from build123d import *

# Parameters (mm, degrees)
BOSS_EXTRUDE1_DEPTH = 7
CUT_EXTRUDE1_DEPTH  = 8
CUT_EXTRUDE2_DEPTH  = 7
SKETCH5_R           = 1.25
CUT_EXTRUDE3_DEPTH  = 8
CUT_EXTRUDE4_DEPTH  = 8


with BuildPart() as part:
    # Sketch1 → Boss-Extrude1 (new body)
    with BuildSketch(Plane.XY):
        Polygon((0, 0), (10, 0), (10, 5), (40, 5), (47.5, -5), (55, -5), (62.5, 5), (55, 12.11693675), (47.5, 12.11693675), (32.5, 12.11693675), (0, 8.5), (0, 5), align=None)
    extrude(amount=BOSS_EXTRUDE1_DEPTH)

    # Sketch3 → Cut-Extrude1 (cut, through all)
    with BuildSketch(Plane.XY.offset(7)):
        Polygon((10, 5), (9.3, 0), (10, 0), align=None)
    extrude(amount=-CUT_EXTRUDE1_DEPTH, mode=Mode.SUBTRACT)

    # Sketch4 → Cut-Extrude2 (cut)
    with BuildSketch(Plane.XY.offset(7)):
        with BuildLine():
            ThreePointArc((51.468681491, 2.792101448), (46.488736675, 7.253317775), (40, 8.865334476))
            ThreePointArc((40, 8.865334476), (39, 7.865334476), (40, 6.865334476))
            ThreePointArc((40, 6.865334476), (45.552771274, 5.485842523), (49.814385807, 1.668132681))
            ThreePointArc((49.814385807, 1.668132681), (51.203518033, 1.402969222), (51.468681491, 2.792101448))
        make_face()
    extrude(amount=-CUT_EXTRUDE2_DEPTH, mode=Mode.SUBTRACT)

    # Sketch5 → Cut-Extrude3 (cut, through all)
    with BuildSketch(Plane.XY.offset(7)):
        with Locations((51.25, -2.5)):
            Circle(SKETCH5_R)
    extrude(amount=-CUT_EXTRUDE3_DEPTH, mode=Mode.SUBTRACT)

    # Sketch6 → Cut-Extrude4 (cut, through all)
    with BuildSketch(Plane.XY.offset(7)):
        Polygon((0, 0), (0.8, 0), (0, 5), align=None)
    extrude(amount=-CUT_EXTRUDE4_DEPTH, mode=Mode.SUBTRACT)


solid = part.part
For this review, take the finished solid that the model builds, in its own axes (mm). A direction names the side the tool comes from. Round coordinates to 2 decimals unless told otherwise and drop trailing zeros. Loops run counter-clockwise (first coordinate to the right, second up) from the corner with the lowest first, then second, coordinate; pieces in that order, holes last. Notation, with made-up numbers: (28.5, 76.25) - (39.5, 76.25) arc R20 ccw to (39.5, 85.25) - close; hole circle Ø7 at (17, 13). An arc over 180 degrees is marked (long way). Answer as CSV lines item,"result".
(1) Consider section B-B on z = 5. Give the boundary of the cut face in (x, y), then the cut area to 3 significant figures.
Checked values:
outline,"(0, 5) - (0.8, 0) - (9.3, 0) - (10, 5) - (40, 5) - (47.5, -5) - (55, -5) - (62.5, 5) - (55, 12.12) - (32.5, 12.12) - (0, 8.5) - close; hole (40, 6.87) arc R11.87 cw to (49.81, 1.67) arc R1 ccw to (51.47, 2.79) arc R13.87 ccw to (40, 8.87) arc R1 ccw to start; hole circle Ø2.5 at (51.25, -2.5)"
area,"522 mm2"
(2) Wall thickness on line 1 (Y direction, x = 51.25, z = 4.75); line 2 (Y direction, x = 38, z = 2.5); line 3 (Y direction, x = 43.5, z = 4.5): over which ranges is each line inside the solid? List them lowest first.
Checked values:
line 1,"y = -5 to -3.75, -1.25 to 1.44, 3.1 to 12.12"
line 2,"y = 5 to 12.12"
line 3,"y = 0.33 to 6.34, 8.42 to 12.12"
(3) Consider section D-D on y = 10.75. Give the boundary of the cut face in (x, z).
Checked values:
outline,"(20.22, 0) - (56.44, 0) - (56.44, 7) - (20.22, 7) - close"
(4) Consider section C-C on x = 36. Give the boundary of the cut face in (y, z), then the cut area to 3 significant figures.
Checked values:
outline,"(5, 0) - (12.12, 0) - (12.12, 7) - (5, 7) - close"
area,"49.8 mm2"
(5) Tool access review of faces 1 (the face through (9.655, 2.535, 3.549)), 2 (the face through (46.57, 7.21, 3.55)), 3 (the face through (44, 12.117, 3)): name each direction out of +Z, -Z, +X, -X, +Y, -Y from which nothing blocks a thin tool from reaching the whole face with its end or side.
Checked values:
face 1,"+Z, -Z, -Y"
face 2,"+Z, -Z"
face 3,"+Z, -Z, +X, -X, +Y"
(6) Mouldability with a two-part tool opening along X and no side actions: class faces 4 (the face through (52.44, -2.12, 3.55)), 5 (the face through (58.698, -0.07, 3.451)), 6 (the face through (16.477, 10.334, 3.451)), 7 (the face through (5, 0, 3)) as +X half, -X half, draft (parallel to the pull), parting line (faces both ways), or undercut.
Checked values:
face 4,"undercut"
face 5,"+X half"
face 6,"-X half"
face 7,"draft"
(7) Consider section A-A on y = -2.5. Give the boundary of the cut face in (x, z) (3 decimals), then the cut area to 4 significant figures.
Checked values:
outline,"(45.625, 0) - (50, 0) - (50, 7) - (45.625, 7) - close; (52.5, 0) - (56.875, 0) - (56.875, 7) - (52.5, 7) - close"
area,"61.25 mm2"
(8) Insertion check: P1, Ø2, axis at x = 3, z = 4, coming from the -Y side; P2, Ø3, axis at x = 13.5, z = 5.5, coming from the -Y side; P3, Ø2, axis at y = 3, z = 4, coming from the +X side. Each pin has a flat end and moves straight along its axis. Give the tip position at first contact, or say it passes through.
Checked values:
P1,"stops at y = 0"
P2,"stops at y = 5"
P3,"stops at x = 61.75"
